The drawing under review shows one solid part. Ordinate dimensions are in mm from its lowest x, y, z. A direction names the side the tool comes from. Give positions to 0.01 mm unless a question says otherwise; leave off trailing zeros. Write each loop counter-clockwise with the first axis right and the second up, starting at its lowest first coordinate (ties: lowest second). Pieces come first, ordered by that corner, then holes. Notation, with made-up numbers: (2.5, 58.5) -> (58.5, 58.5) arc R20 cw to (58.5, 97.5) -> close; hole circle Ø3 at (65.25, 32.5). An arc over 180 degrees is marked (long way). Use CSV: the item, a comma, the result in double quotes.
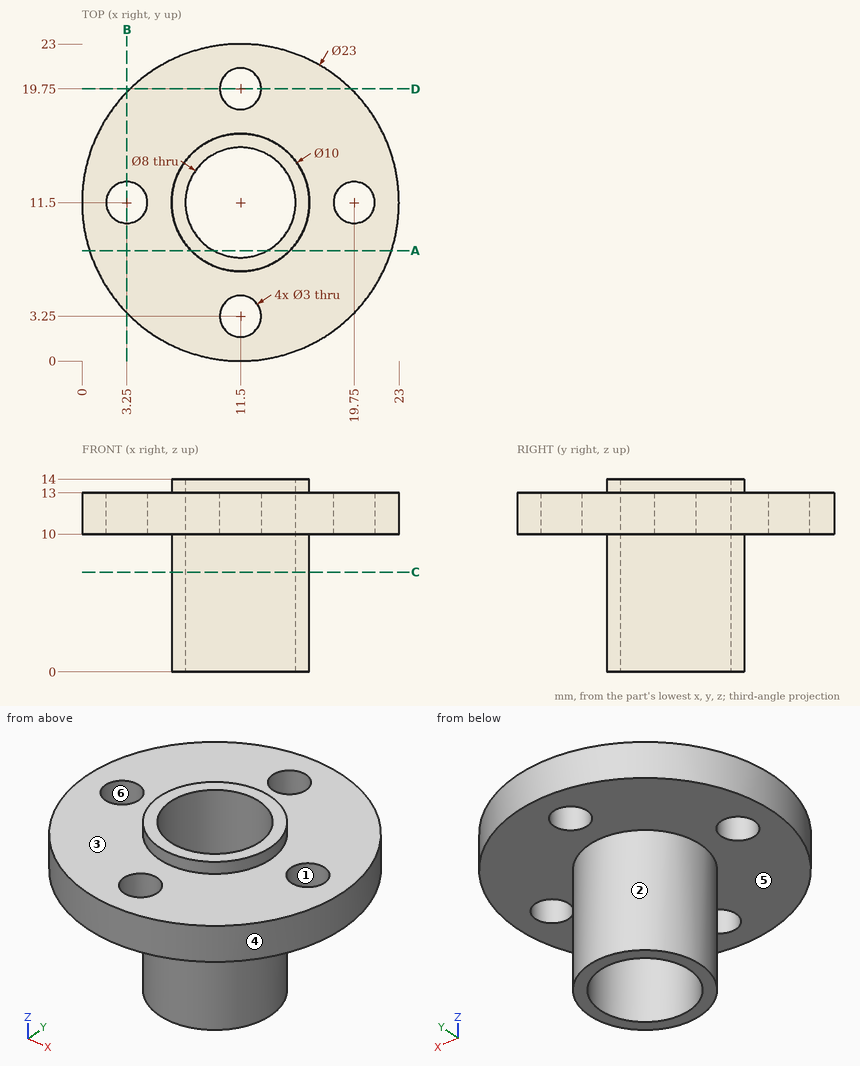
(1) Clearance check with flat-ended pins moving along their axes: pin 1 (11.5 mm diameter, centred on x = 14, y = 7, fed in from +Z); pin 2 (5 mm diameter, centred on x = 11, z = 4.5, fed in from +Y); pin 3 (6 mm diameter, centred on x = 4.5, z = 6, fed in from +Y); pin 4 (4 mm diameter, centred on x = 19.75, y = 11.5, fed in from -Z). State where each tip first meets the part, or that it passes through.
Established:
pin 1,"stops at z = 14"
pin 2,"stops at y = 16.5"
pin 3,"stops at y = 14.5"
pin 4,"stops at z = 10"
(2) Take a section at A-A (y = 8). Write out the cut boundary in (x, z), then the cut area to 3 significant figures.
Established:
outline,"(0.55, 10) -> (7.93, 10) -> (7.93, 0) -> (9.56, 0) -> (9.56, 14) -> (7.93, 14) -> (7.93, 13) -> (0.55, 13) -> close; (13.44, 0) -> (15.07, 0) -> (15.07, 10) -> (22.45, 10) -> (22.45, 13) -> (15.07, 13) -> (15.07, 14) -> (13.44, 14) -> close"
area,"90.1 mm2"
(3) Take a section at B-B (x = 3.25). Write out the cut boundary in (y, z), then the cut area to 3 significant figures.
Established:
outline,"(3.49, 10) -> (10, 10) -> (10, 13) -> (3.49, 13) -> close; (13, 10) -> (19.51, 10) -> (19.51, 13) -> (13, 13) -> close"
area,"39.1 mm2"
(4) Take a section at C-C (z = 7.25). Write out the cut boundary in (x, y).
Established:
outline,"circle Ø10 at (11.5, 11.5); hole circle Ø8 at (11.5, 11.5)"
(5) Mouldability with a two-part tool opening along Y and no side actions: class the marked faces 4, 5 and 6 as +Y half, -Y half, draft (parallel to the pull), parting line (faces both ways), or undercut.
Established:
face 4,"parting line"
face 5,"draft"
face 6,"undercut"
(6) Tool access review of the marked faces 1, 2 and 3: name each direction out of +Z, -Z, +X, -X, +Y, -Y from which nothing blocks a thin tool from reaching the whole face with its end or side.
Established:
face 1,"+Z, -Z"
face 2,"-Z"
face 3,"+Z"
(7) For line 1 along Y through (x, z) = (11.5, 12); line 2 along Z through (x, y) = (3, 8.25); line 3 along X through (y, z) = (13.5, 3), list the stretches that pass through material, from the lowest coordinate up. Write a range as [from, to].
Established:
line 1,"y = [0, 1.75], [4.75, 7.5], [15.5, 18.25], [21.25, 23]"
line 2,"z = [10, 13]"
line 3,"x = [6.92, 8.04], [14.96, 16.08]"
